Design review of the part built by this model. Coordinates are the model's own, in mm. Face numbers are marked on the shaded views. Give positions to 0.01 mm unless a question says otherwise; leave off trailing zeros. Write each loop counter-clockwise with the first axis right and the second up, starting at its lowest first coordinate (ties: lowest second). Pieces come first, ordered by that corner, then holes. Notation, with made-up numbers: M 88,80.25 L 137,80.25 A6 ccw 137,90.25 Z; hole C -13.5,27.5 d3. An arc over 180 degrees is marked long. One line per item, written item: value. Start each with the question number.
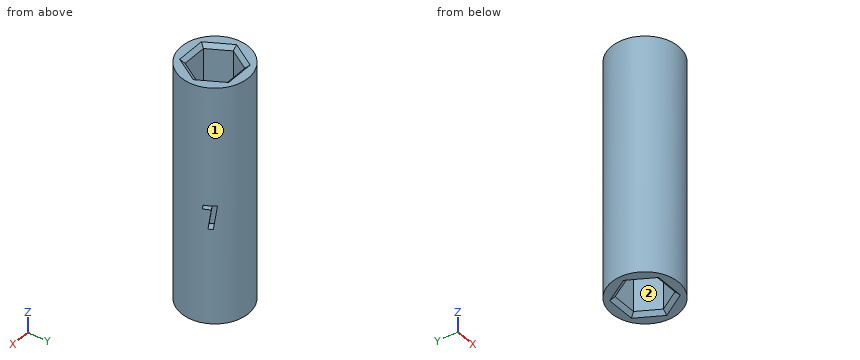
```python
from build123d import *

# Parameters (mm, degrees)
SKETCH1_W          = 4.5
SKETCH1_H          = 32.11709914
CUT_EXTRUDE1_DEPTH = 7
CUT_EXTRUDE2_DEPTH = 7
CHAMFER1_SIZE      = 0.5
CUT_EXTRUDE3_DEPTH = 1


with BuildPart() as part:
    # Sketch1 → Revolve-Thin1 (revolve)
    with BuildSketch(Plane(origin=(0, 0, 0), x_dir=(1, 0, 0), z_dir=(0, 1, 0))):
        with Locations((2.25, 33.55854957)):
            Rectangle(SKETCH1_W, SKETCH1_H)
    revolve(axis=Axis((0, 0, 0), (0, 0, -1)))

    # Sketch2 → Cut-Extrude1 (cut)
    with BuildSketch(Plane.XY.offset(-17.5)):
        Polygon((1.610807251, 2.79), (-1.610807251, 2.79), (-3.221614502, 0), (-1.610807251, -2.79), (1.610807251, -2.79), (3.221614502, 0), align=None)
    extrude(amount=-CUT_EXTRUDE1_DEPTH, mode=Mode.SUBTRACT)

    # Sketch3 → Cut-Extrude2 (cut)
    with BuildSketch(Plane(origin=(0, 0, -49.61709914), x_dir=(-1, 0, 0), z_dir=(0, 0, -1))):
        Polygon((1.610807251, 2.79), (-1.610807251, 2.79), (-3.221614502, 0), (-1.610807251, -2.79), (1.610807251, -2.79), (3.221614502, 0), align=None)
    extrude(amount=-CUT_EXTRUDE2_DEPTH, mode=Mode.SUBTRACT)

    # Chamfer1
    chamfer1_edges = [part.edges().sort_by_distance(p)[0] for p in [
        (2.416210877, 1.395, -17.5),
        (0, 2.79, -17.5),
        (-2.416210877, 1.395, -17.5),
        (-2.416210877, -1.395, -17.5),
        (0, -2.79, -17.5),
        (2.416210877, -1.395, -17.5),
        (-2.416210877, 1.395, -49.61709914),
        (0, 2.79, -49.61709914),
        (2.416210877, 1.395, -49.61709914),
        (2.416210877, -1.395, -49.61709914),
        (0, -2.79, -49.61709914),
        (-2.416210877, -1.395, -49.61709914),
    ]]
    chamfer(chamfer1_edges, length=CHAMFER1_SIZE)

    # Sketch4 → Cut-Extrude3 (cut)
    with BuildSketch(Plane(origin=(3.897114317, 2.25, 0), x_dir=(0, 0, -1), z_dir=(0.866025404, 0.5, 0))):
        Polygon((36.73354957, 0.409595353), (36.73354957, -0.166636619), (34.087716237, 0.204797676), (34.087716237, -0.773397436), (33.55854957, -0.704707532), (33.55854957, 0.854807692), align=None)
    extrude(amount=-CUT_EXTRUDE3_DEPTH, mode=Mode.SUBTRACT)


solid = part.part
```
Q1. Take a section at B-B, the plane y = -2. Give the boundary of the cut face in (x, z), then the cut area to 3 significant figures.
Q2. Take a section at C-C, the plane z = -25. Give the boundary of the cut face in (x, y), then the cut area to 3 significant figures.
Q3. Wall thickness on line 1 (Y direction, x = -0.25, z = -27.5); line 2 (Z direction, x = 0.5, y = 0.5); line 3 (Y direction, x = 1, z = -20.5): over which ranges is each line inside the solid? List them lowest first. Write a range as from..to.
Q4. Take a section at A-A, the plane x = 0. Give the boundary of the cut face in (y, z).
Q5. The part is to be moulded in two halves that separate along X. For the marked faces 1 and 2, say which applies: pulls with the +X half, pulls with the -X half, needs draft (parallel to the pull), parting line crosses it, or undercut.
Q6. For P1, Ø2, axis at x = -0.5, y = 1, coming from the -Z side; P2, Ø1.5, axis at y = 1, z = -28.5, coming from the +X side; P3, Ø1.5, axis at y = 1.5, z = -31, coming from the +X side; P4, Ø3.5, axis at x = -0.5, z = -45, coming from the +Y side, all flat-tipped, find the tip position at first contact; note any pin that passes through.
Results list:
1. outline: M -4.03,-49.62 L -2.64,-49.62 L -2.07,-49.12 L -2.07,-42.62 L 2.07,-42.62 L 2.07,-49.12 L 2.64,-49.62 L 4.03,-49.62 L 4.03,-17.5 L 2.64,-17.5 L 2.07,-18 L 2.07,-24.5 L -2.07,-24.5 L -2.07,-18 L -2.64,-17.5 L -4.03,-17.5 Z
1. area: 200 mm^2
2. outline: C 0,0 d9
2. area: 63.6 mm^2
3. line 1: y = -4.49..4.49
3. line 2: z = -42.62..-24.5
3. line 3: y = -4.39..-2.79, 2.79..4.39
4. outline: M -4.5,-49.62 L -3.29,-49.62 L -2.79,-49.12 L -2.79,-42.62 L 2.79,-42.62 L 2.79,-49.12 L 3.29,-49.62 L 4.5,-49.62 L 4.5,-17.5 L 3.29,-17.5 L 2.79,-18 L 2.79,-24.5 L -2.79,-24.5 L -2.79,-18 L -3.29,-17.5 L -4.5,-17.5 Z
5. face 1: parting line crosses it
5. face 2: undercut
6. P1: stops at z = -42.62
6. P2: stops at x = 4.49
6. P3: stops at x = 4.44
6. P4: stops at y = 4.5
